Here's the drawing with two shaded views (mm, measured from the low corner). I have some questions. A direction names the side the tool comes from. Give positions to 0.01 mm unless a question says otherwise; leave off trailing zeros. Write each loop counter-clockwise with the first axis right and the second up, starting at its lowest first coordinate (ties: lowest second). Pieces come first, ordered by that corner, then holes. Notation, with made-up numbers: M 28.5,61.5 L 43.5,61.5 A24 cw 43.5,84.5 Z; hole C -4,61.5 d2. An arc over 180 degrees is marked long. Use one line per item in the form item = value.
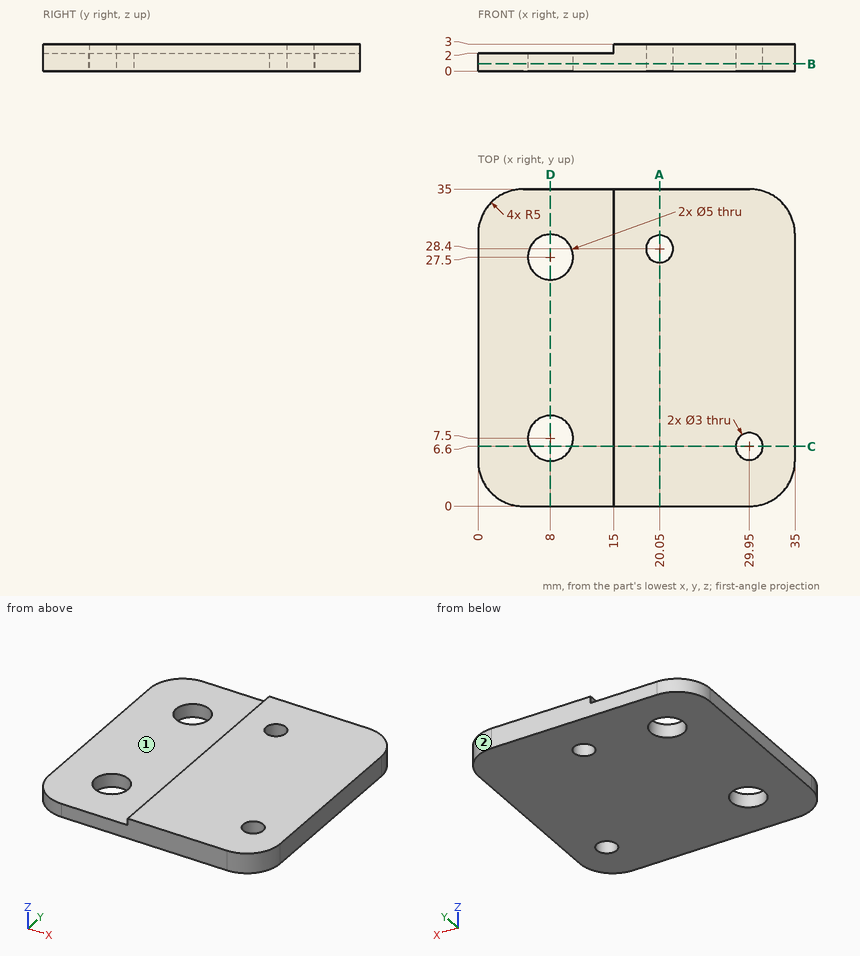
1) I want a section at C-C, the plane y = 6.6. Please give me the cut outline in (x, z), plus the area to 3 significant figures.
Checked values:
outline = M 0,0 L 5.67,0 L 5.67,2 L 0,2 Z; M 10.33,0 L 28.45,0 L 28.45,3 L 15,3 L 15,2 L 10.33,2 Z; M 31.45,0 L 35,0 L 35,3 L 31.45,3 Z
area = 71.7 mm2
2) I want a section at D-D, the plane x = 8. Please give me the cut outline in (y, z).
Checked values:
outline = M 0,0 L 5,0 L 5,2 L 0,2 Z; M 10,0 L 25,0 L 25,2 L 10,2 Z; M 30,0 L 35,0 L 35,2 L 30,2 Z
3) If I drill on L1, parallel to Y at x = 8, z = 0.65; L2, parallel to Y at x = 29.95, z = 2.3; L3, parallel to Z at x = 4, y = 20, over which ranges is the centre line in solid material (lowest first)?
Checked values:
L1 = 0 to 5, 10 to 25, 30 to 35
L2 = 0 to 5.1, 8.1 to 35
L3 = 0 to 2
4) I want a section at A-A, the plane x = 20.05. Please give me the cut outline in (y, z).
Checked values:
outline = M 0,0 L 26.9,0 L 26.9,3 L 0,3 Z; M 29.9,0 L 35,0 L 35,3 L 29.9,3 Z
5) For the marked faces 1 and 2, which set-ups out of +Z, -Z, +X, -X, +Y, -Y let a thin tool reach every point of the face, with its end or its side?
Checked values:
face_1 = +Z, -X, +Y, -Y
face_2 = +Z, -Z, +X, +Y
6) I want a section at B-B, the plane z = 0.8. Please give me the cut outline in (x, y), plus the area to 3 significant figures.
Checked values:
outline = M 0,5 A5 ccw 5,0 L 30,0 A5 ccw 35,5 L 35,30 A5 ccw 30,35 L 5,35 A5 ccw 0,30 Z; hole C 8,7.5 d5; hole C 8,27.5 d5; hole C 20.05,28.4 d3; hole C 29.95,6.6 d3
area = 1,150 mm2
7) For pin 1 Ø10 at (x, y) = (4, 14) entering from -Z; pin 2 Ø0.8 at (y, z) = (24.5, 2.5) entering from -X; pin 3 Ø12 at (x, y) = (6.5, 24.5) entering from +Z; pin 4 Ø3 at (x, y) = (8, 7.5) entering from +Z, each with a flat end and sliding along its axis, tell me the tip position at first contact or that it passes through.
Checked values:
pin_1 = 0
pin_2 = 15
pin_3 = 2
pin_4 = through
